The model under review builds one solid part; all positions refer to its coordinate system, in mm. Face numbers are marked on the shaded views. A direction names the side the tool comes from. Give positions to 0.01 mm unless a question says otherwise; leave off trailing zeros. Order: outer loops, then holes, each group sorted by start corner. A loop starts at its lowest first (then second) coordinate and runs counter-clockwise, first axis right, second up. Notation, with made-up numbers: (36, 6) - (81, 6) arc R30 cw to (81, 34) - close; hole circle Ø9 at (-25, 43). An arc over 180 degrees is marked (long way). Use CSV: the item, a comma, the result in double quotes. Start each with the question number.
1. Take a section at A-A, the plane y = 239. State the section outline as (x, z) points.
2. Machinability: for the marked faces 1 and 2, which of the approach directions +Z, -Z, +X, -X, +Y, -Y give a long, thin tool a straight path to every point of the face, cutting with its end or side? Answer none if there is none.
3. Take a section at D-D, the plane y = 136. State the section outline as (x, z) points.
4. Take a section at B-B, the plane x = 70. State the section outline as (y, z) points (1 decimal).
5. For pin 1 (1.5 mm diameter, centred on x = -4, z = 138.5, fed in from -Y); pin 2 (15.5 mm diameter, centred on x = 420, y = 170.5, fed in from -Z); pin 3 (2 mm diameter, centred on y = 316.5, z = -228.5, fed in from +X), all flat-tipped, find the tip position at first contact; note any pin that passes through.
6. Draft analysis for pull direction Y (two halves, no side actions). For the marked faces 3, 4 and 5, state which applies: released by +Y, released by -Y, zero draft, split by the parting line, or undercut.
7. To check wall thickness, follow line 1 (Y direction, x = 156.5, z = -221.5) (1 decimal); line 2 (Z direction, x = 418, y = 408); line 3 (Z direction, x = 359, y = 136). State the ranges of each line that lie inside material, in increasing order. Write a range as [from, to].
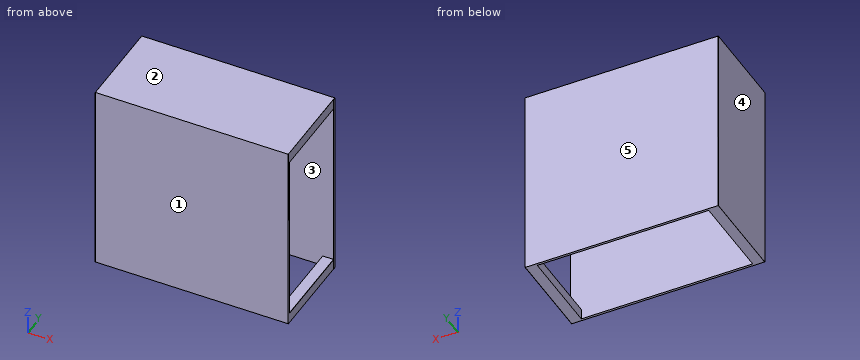
```python
from build123d import *

# Parameters (mm, degrees)
BOSS_EXTRUDE1_DEPTH  = 11.1125
SKETCH1_5_W          = 50.8
SKETCH1_5_H          = 50.8
BOSS_EXTRUDE3_DEPTH  = 417.5125
SKETCH1_6_W          = 50.8
SKETCH1_6_H          = 50.8
BOSS_EXTRUDE4_DEPTH  = 417.5125
SKETCH1_7_W          = 50.8
SKETCH1_7_H          = 50.8
BOSS_EXTRUDE5_DEPTH  = 417.5125
SKETCH1_8_W          = 50.8
SKETCH1_8_H          = 50.8
BOSS_EXTRUDE6_DEPTH  = 417.5125
SKETCH2_W            = 915.815141898
SKETCH2_H            = 914.4
BOSS_EXTRUDE8_DEPTH  = 11.1125
SKETCH3_W            = 914.440346881
SKETCH3_H            = 428.625
BOSS_EXTRUDE9_DEPTH  = 0.4375
SKETCH4_W            = 814.910119316
SKETCH4_H            = 406.4
BOSS_EXTRUDE13_DEPTH = 0.4375
BOSS_EXTRUDE21_DEPTH = 0.4375


with BuildPart() as part:
    # Sketch1 → Boss-Extrude1 (new body)
    with BuildSketch(Plane(origin=(0, 0, 0), x_dir=(1, 0, 0), z_dir=(0, 1, 0))):
        Polygon((-406.4, 406.4), (-457.2, 406.4), (-457.2, -406.4), (-406.4, -406.4), (-406.4, -457.2), (406.4, -457.2), (406.4, -406.4), (457.2, -406.4), (457.2, 406.4), (406.4, 406.4), (406.4, 457.2), (-406.4, 457.2), align=None)
    extrude(amount=BOSS_EXTRUDE1_DEPTH)

    # Sketch1<5> → Boss-Extrude3 (add)
    with BuildSketch(Plane(origin=(0, 0, 0), x_dir=(1, 0, 0), z_dir=(0, 1, 0))):
        with Locations((431.8, -431.8)):
            Rectangle(SKETCH1_5_W, SKETCH1_5_H)
    extrude(amount=BOSS_EXTRUDE3_DEPTH)

    # Sketch1<6> → Boss-Extrude4 (add)
    with BuildSketch(Plane(origin=(0, 0, 0), x_dir=(1, 0, 0), z_dir=(0, 1, 0))):
        with Locations((-431.8, -431.8)):
            Rectangle(SKETCH1_6_W, SKETCH1_6_H)
    extrude(amount=BOSS_EXTRUDE4_DEPTH)

    # Sketch1<7> → Boss-Extrude5 (add)
    with BuildSketch(Plane(origin=(0, 0, 0), x_dir=(1, 0, 0), z_dir=(0, 1, 0))):
        with Locations((431.8, 431.8)):
            Rectangle(SKETCH1_7_W, SKETCH1_7_H)
    extrude(amount=BOSS_EXTRUDE5_DEPTH)

    # Sketch1<8> → Boss-Extrude6 (add)
    with BuildSketch(Plane(origin=(0, 0, 0), x_dir=(1, 0, 0), z_dir=(0, 1, 0))):
        with Locations((-431.8, 431.8)):
            Rectangle(SKETCH1_8_W, SKETCH1_8_H)
    extrude(amount=BOSS_EXTRUDE6_DEPTH)

    # Sketch2 → Boss-Extrude8 (add)
    with BuildSketch(Plane(origin=(0, 417.5125, 0), x_dir=(1, 0, 0), z_dir=(0, 1, 0))):
        with Locations((0.707570949, 0)):
            Rectangle(SKETCH2_W, SKETCH2_H)
    extrude(amount=BOSS_EXTRUDE8_DEPTH)

    # Sketch3 → Boss-Extrude9 (add)
    with BuildSketch(Plane.XY.offset(457.2)):
        with Locations((0.020173441, 214.3125)):
            Rectangle(SKETCH3_W, SKETCH3_H)
    extrude(amount=BOSS_EXTRUDE9_DEPTH)

    # Sketch4 → Boss-Extrude13 (add)
    with BuildSketch(Plane(origin=(457.2, 0, 0), x_dir=(0, 0, -1), z_dir=(1, 0, 0))):
        Polygon((-457.2, 428.625), (-457.6375, 0), (457.580376967, -0.934168145), (458.017876967, 427.690831855), align=None)
        with Locations((1.055059658, 214.3125)):
            Rectangle(SKETCH4_W, SKETCH4_H, mode=Mode.SUBTRACT)
    extrude(amount=BOSS_EXTRUDE13_DEPTH)

    # Sketch10 → Boss-Extrude21 (add)
    with BuildSketch(Plane.ZY.offset(457.2)):
        Polygon((-457.2, 428.625), (-457.580376967, -0.934168145), (456.953407178, -1.743992758), (457.333784145, 427.815175387), align=None)
    extrude(amount=BOSS_EXTRUDE21_DEPTH)


solid = part.part
```
Determined:
1,outline,"(-457.64, -457.37) - (-457.2, -457.37) - (-457.2, -457.2) - (-406.4, -457.2) - (-406.4, -406.4) - (-457.2, -406.4) - (-457.2, 406.4) - (-406.4, 406.4) - (-406.4, 457.2) - (406.4, 457.2) - (406.4, 406.4) - (457.64, 406.4) - (457.64, 457.39) - (457.24, 457.39) - (457.24, 457.64) - (-457.2, 457.64) - (-457.2, 457.17) - (-457.64, 457.17) - close; (406.4, -457.2) - (457.2, -457.2) - (457.2, -457.83) - (457.64, -457.83) - (457.64, -408.51) - (457.2, -408.51) - (457.2, -406.4) - (406.4, -406.4) - close"
2,face 1,"+Z, -Z, -Y"
2,face 2,"+Z, +X, -X, +Y, -Y"
3,outline,"(-457.64, -457.46) - (-457.2, -457.46) - (-457.2, -457.2) - (-406.4, -457.2) - (-406.4, -406.4) - (-457.2, -406.4) - (-457.2, 406.4) - (-406.4, 406.4) - (-406.4, 457.2) - (406.4, 457.2) - (406.4, 406.4) - (457.64, 406.4) - (457.64, 457.5) - (457.24, 457.5) - (457.24, 457.64) - (-457.2, 457.64) - (-457.2, 457.08) - (-457.64, 457.08) - close; (406.4, -457.2) - (457.2, -457.2) - (457.2, -457.72) - (457.64, -457.72) - (457.64, -408.51) - (457.2, -408.51) - (457.2, -406.4) - (406.4, -406.4) - close"
4,outline,"(0, -457.2) - (11.1, -457.2) - (11.1, 457.2) - (417.5, 457.2) - (417.5, -457.2) - (428.6, -457.2) - (428.6, 457.6) - (0, 457.6) - close"
5,pin 1,"stops at y = 0"
5,pin 2,"stops at z = -457.2"
5,pin 3,"stops at x = -457.2"
6,face 3,"undercut"
6,face 4,"zero draft"
6,face 5,"released by +Y"
7,line 1,"y = [0, 11.1], [417.5, 428.6]"
7,line 2,"z = [-457.2, -406.4], [406.4, 457.64]"
7,line 3,"z = [457.2, 457.64]"
